```python
from build123d import *

# Parameters (mm, degrees)
F1_DEPTH = 8
F2_R     = 3.5
F3_DEPTH = 4.5
F4_R     = 2
F5_R     = 2
F6_DEPTH = 25


with BuildPart() as f1:
    # F0 (on Top) → F1 (new body)
    with BuildSketch(Plane.XY):
        with BuildLine():
            Line((-2.498805, 8), (-10, 8))
            Line((-10, 8), (-10, 0))
            Line((-10, 0), (10, 0))
            Line((10, 0), (10, 8))
            Line((10, 8), (2.379432, 8))
            Line((2.379432, 8), (2.496949, 5.623472))
            ThreePointArc((2.496949, 5.623472), (0.023112, 3.000107), (-2.498805, 5.577284))
            Line((-2.498805, 5.577284), (-2.498805, 8))
        make_face()
    extrude(amount=F1_DEPTH)

    # F2 (on face) → F3 (cut)
    with BuildSketch(Plane.XZ):
        with Locations((6, 4)):
            Circle(F2_R)
        with Locations((-6, 4)):
            Circle(F2_R)
    extrude(amount=-F3_DEPTH, mode=Mode.SUBTRACT)

    # F4 (on face) + F5 (on face) → F6 (cut)
    with BuildSketch(Plane.XZ.offset(-4.5)):
        with Locations((-6, 4)):
            Circle(F4_R)
    with BuildSketch(Plane.XZ.offset(-4.5)):
        with Locations((6, 4)):
            Circle(F5_R)
    extrude(amount=-F6_DEPTH, mode=Mode.SUBTRACT)


solid = f1.part
```
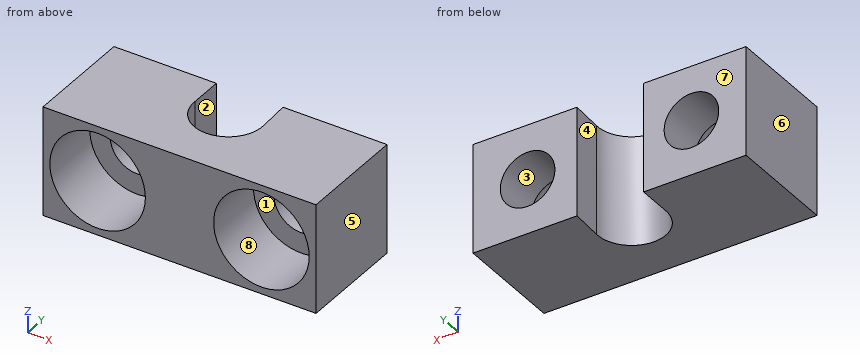
Check sheet for the modelled part. Datum: model origin and axes. Units: mm. Face numbers are marked on the shaded views. A direction names the side the tool comes from. Give positions to 0.01 mm unless a question says otherwise; leave off trailing zeros. Loops run counter-clockwise (first coordinate to the right, second up) from the corner with the lowest first, then second, coordinate; pieces in that order, holes last. Notation, with made-up numbers: M 18.5,-3.75 L 35.5,-3.75 A33 ccw 35.5,25.25 Z; hole C 39.5,48.25 d3. An arc over 180 degrees is marked long. Answer in a Markdown table with one row per item.
1) Mould release check, pull along X, two halves, no side actions. Record for the marked faces 6, 7 and 8: released by +X, released by -X, zero draft, split by the parting line, or undercut.
Solutions:
| item | result |
|---|---|
| face 6 | released by -X |
| face 7 | zero draft |
| face 8 | undercut |
2) Cross-section at A-A (x = 6). Enter the section's corners in (y, z), plus the area to 3 significant figures.
Solutions:
| item | result |
|---|---|
| outline | M 0,0 L 8,0 L 8,2 L 4.5,2 L 4.5,0.5 L 0,0.5 Z; M 0,7.5 L 4.5,7.5 L 4.5,6 L 8,6 L 8,8 L 0,8 Z |
| area | 18.5 mm^2 |
3) Depth check by flat-ended pin: pin 1 (2 mm diameter, centred on x = 6, z = 5.5, fed in from -Y); pin 2 (4 mm diameter, centred on x = 0, z = 6.5, fed in from +Y). Enter the tip coordinate at first touch or a pass-through.
Solutions:
| item | result |
|---|---|
| pin 1 | stops at y = 4.5 |
| pin 2 | stops at y = 4 |
4) Thickness scan on line 1 (Z direction, x = 6, y = 6.25); line 2 (Z direction, x = 6, y = 2.45); line 3 (X direction, y = 6.5, z = 4.25). Record the ranges inside material, lowest first.
Solutions:
| item | result |
|---|---|
| line 1 | z = 0 to 2, 6 to 8 |
| line 2 | z = 0 to 0.5, 7.5 to 8 |
| line 3 | x = -10 to -7.98, -4.02 to -2.5, 2.45 to 4.02, 7.98 to 10 |
5) Cross-section at B-B (z = 4). Enter the section's corners in (x, y), plus the area to 3 significant figures.
Solutions:
| item | result |
|---|---|
| outline | M -10,0 L -9.5,0 L -9.5,4.5 L -8,4.5 L -8,8 L -10,8 Z; M -4,4.5 L -2.5,4.5 L -2.5,0 L 2.5,0 L 2.5,4.5 L 4,4.5 L 4,8 L 2.38,8 L 2.5,5.62 A2.5 cw long -2.5,5.58 L -2.5,8 L -4,8 Z; M 8,4.5 L 9.5,4.5 L 9.5,0 L 10,0 L 10,8 L 8,8 Z |
| area | 46.8 mm^2 |
6) Cross-section at C-C (y = 5). Enter the section's corners in (x, z).
Solutions:
| item | result |
|---|---|
| outline | M -10,0 L -2.45,0 L -2.45,8 L -10,8 Z; M 2.45,0 L 10,0 L 10,8 L 2.45,8 Z; hole C -6,4 d4; hole C 6,4 d4 |
7) Tool access check on the marked faces 1, 2, 3, 4 and 5. Record the directions out of +Z, -Z, +X, -X, +Y, -Y that give a thin tool (end or side, any length) a straight path to the whole face; none if there is none.
Solutions:
| item | result |
|---|---|
| face 1 | -Y |
| face 2 | +Z, -Z, +Y |
| face 3 | +Y, -Y |
| face 4 | +Z, -Z |
| face 5 | +Z, -Z, +X, +Y, -Y |
8) Cross-section at D-D (y = 3.25). Enter the section's corners in (x, z).
Solutions:
| item | result |
|---|---|
| outline | M -10,0 L -1.09,0 L -1.09,8 L -10,8 Z; M 1.09,0 L 10,0 L 10,8 L 1.09,8 Z; hole C -6,4 d7; hole C 6,4 d7 |
